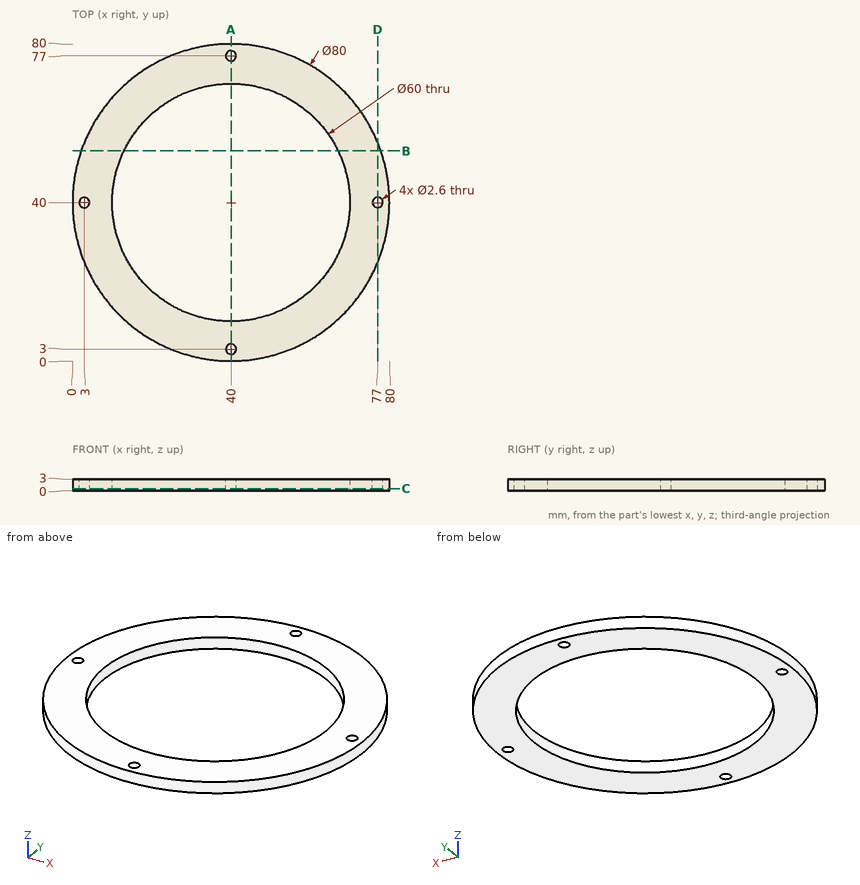
Check sheet for the drawn part. Datum: minimum x, y, z corner. Units: mm. Round coordinates to 2 decimals unless told otherwise and drop trailing zeros. Order: outer loops, then holes, each group sorted by start corner. A loop starts at its lowest first (then second) coordinate and runs counter-clockwise, first axis right, second up. Notation, with made-up numbers: M -33.75,10.25 L -11.75,10.25 A17 ccw -11.75,23.25 Z; hole C 79,81 d2. An arc over 180 degrees is marked long. Write each question's results on one line, items separated by ' | '. Start each with the question number.
1. Cross-section at B-B on y = 53. Record the boundary of the cut face in (x, z), plus the area to 3 significant figures.
2. Material ranges on L1, parallel to X at y = 39.5, z = 0.7; L2, parallel to X at y = 25.5, z = 1.8; L3, parallel to Y at x = 28.5, z = 1.1, recorded low to high. Write a range as from..to.
3. Cross-section at D-D on x = 77. Record the boundary of the cut face in (y, z).
4. Cross-section at A-A on x = 40. Record the boundary of the cut face in (y, z).
5. Cross-section at C-C on z = 0.6. Record the boundary of the cut face in (x, y).
6. Go/stop test with flat-tipped pins: P1, Ø1.6, axis at x = 40, y = 3, coming from the +Z side; P2, Ø1.5, axis at x = 67.5, z = 1, coming from the -Y side. Record where each tip stops, or that it passes through.
Resolved:
1) outline: M 2.17,0 L 12.96,0 L 12.96,3 L 2.17,3 Z; M 67.04,0 L 77.83,0 L 77.83,3 L 67.04,3 Z | area: 64.7 mm2
2) L1: 0..1.8, 4.2..10, 70..75.8, 78.2..80 | L2: 2.72..13.74, 66.26..77.28 | L3: 1.69..12.29, 67.71..78.31
3) outline: M 24.8,0 L 38.7,0 L 38.7,3 L 24.8,3 Z; M 41.3,0 L 55.2,0 L 55.2,3 L 41.3,3 Z
4) outline: M 0,0 L 1.7,0 L 1.7,3 L 0,3 Z; M 4.3,0 L 10,0 L 10,3 L 4.3,3 Z; M 70,0 L 75.7,0 L 75.7,3 L 70,3 Z; M 78.3,0 L 80,0 L 80,3 L 78.3,3 Z
5) outline: C 40,40 d80; hole C 3,40 d2.6; hole C 40,40 d60; hole C 40,3 d2.6; hole C 40,77 d2.6; hole C 77,40 d2.6
6) P1: through | P2: y = 10.26
